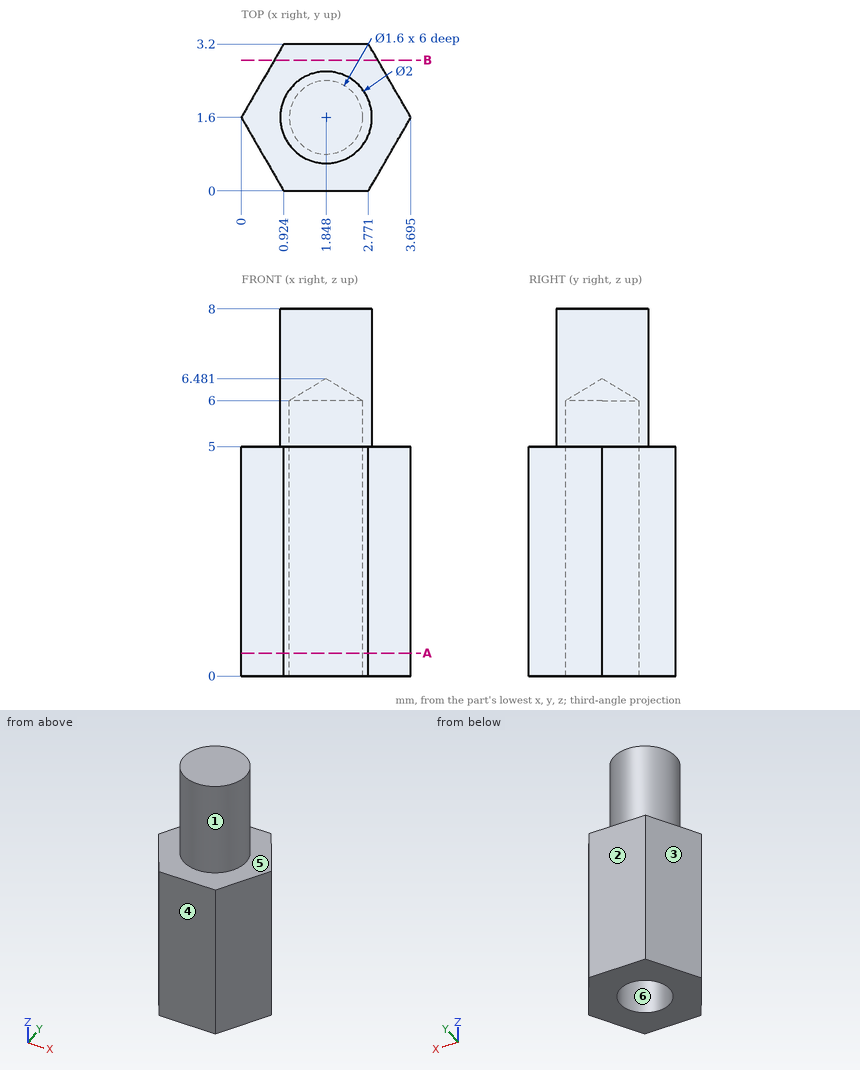
Verification items for this drawing (mm, ordinates from the low corner). A direction names the side the tool comes from. Give positions to 0.01 mm unless a question says otherwise; leave off trailing zeros. Write each loop counter-clockwise with the first axis right and the second up, starting at its lowest first coordinate (ties: lowest second). Pieces come first, ordered by that corner, then holes. Notation, with made-up numbers: (74.5, 25.25) -> (119.5, 25.25) arc R3 cw to (119.5, 30.25) -> close; hole circle Ø5 at (-1.5, -32.5). An arc over 180 degrees is marked (long way). Use CSV: the item, a comma, the result in double quotes. Start each with the question number.
Q1. Cross-section at A-A on z = 0.5. Enter the section's corners in (x, y) (1 decimal).
Q2. Cross-section at B-B on y = 2.85. Enter the section's corners in (x, z).
Q3. Tool access check on the marked faces 1 and 2. Record the directions out of +Z, -Z, +X, -X, +Y, -Y that give a thin tool (end or side, any length) a straight path to the whole face; none if there is none.
Q4. Release check for a two-part mould opening along Y. For the marked faces 3, 4, 5 and 6 record: +Y half, -Y half, draft (parallel to the pull), parting line (faces both ways), or undercut.
Q5. Scan lines: line 1 along Z through (x, y) = (2.7, 2.5); line 2 along X through (y, z) = (1.75, 4.75) (1 decimal); line 3 along Y through (x, z) = (1.8, 7). Record each from-to range of solid material in increasing order.
Working result:
1,outline,"(0, 1.6) -> (0.9, 0) -> (2.8, 0) -> (3.7, 1.6) -> (2.8, 3.2) -> (0.9, 3.2) -> close; hole circle Ø1.6 at (1.8, 1.6)"
2,outline,"(0.72, 0) -> (2.97, 0) -> (2.97, 5) -> (0.72, 5) -> close"
3,face 1,"+Z"
3,face 2,"+Z, -Z, +X, -X, +Y"
4,face 3,"+Y half"
4,face 4,"-Y half"
4,face 5,"draft"
4,face 6,"undercut"
5,line 1,"z = 0 to 5"
5,line 2,"x = 0.1 to 1.1, 2.6 to 3.6"
5,line 3,"y = 0.6 to 2.6"
